The figure shows three views and two pictorial views of one solid part (mm, origin at its lowest corner). Answer the questions. A direction names the side the tool comes from. Coordinates: 2 decimals unless noted, no trailing zeros. Loops run counter-clockwise (first coordinate to the right, second up) from the corner with the lowest first, then second, coordinate; pieces in that order, holes last. Notation, with made-up numbers: M 85.25,68 L 134.25,68 A21 cw 134.25,78 Z; hole C 56,65 d8. An arc over 180 degrees is marked long. One line per item, written item: value. Start each with the question number.
1. The part is cut by section C-C (x = 11.5). Write down the section's boundary in (y, z), then the cut area to 3 significant figures.
2. The part is cut by section B-B (y = 9.5). Write down the section's boundary in (x, z).
3. The part is cut by section A-A (z = 1.45). Write down the section's boundary in (x, y), then the cut area to 3 significant figures.
4. Flat-ended cylindrical pins translate along their axes: pin 1 (2 mm diameter, centred on x = 13.5, z = 4, fed in from +Y); pin 2 (2.5 mm diameter, centred on y = 6.5, z = 3.5, fed in from -X). Find the tip coordinate at first contact, or state that the pin passes through.
5. For the marked faces 1 and 2, determine the directions among +Z, -Z, +X, -X, +Y, -Y from which every point of the face is accessible in a straight line to the end or side of a thin tool.
6. Consider probe 1 along Y at (x, z) = (8, 4.75); probe 2 along X at (y, z) = (3, 2.6); probe 3 along Y at (x, z) = (16, 0.35). Determine where each line is inside the solid, lowest interval first.
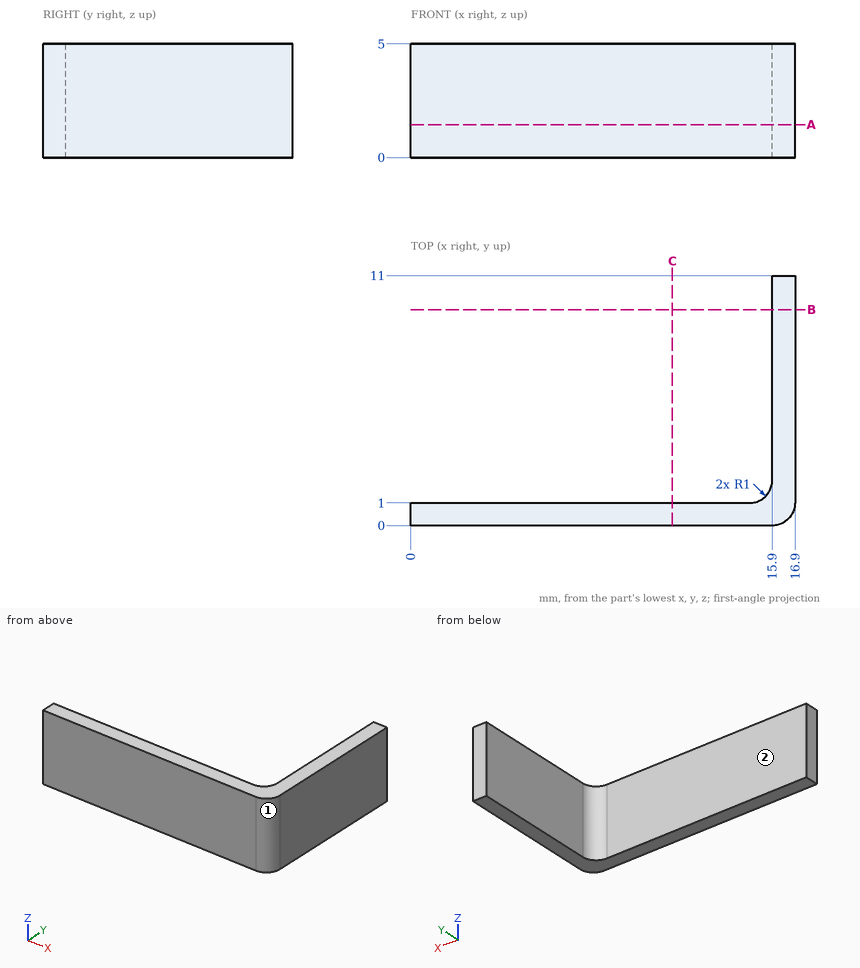
Answer block:
1. outline: M 0,0 L 1,0 L 1,5 L 0,5 Z
1. area: 5.00 mm2
2. outline: M 15.9,0 L 16.9,0 L 16.9,5 L 15.9,5 Z
3. outline: M 0,0 L 15.9,0 A1 ccw 16.9,1 L 16.9,11 L 15.9,11 L 15.9,2 A1 cw 14.9,1 L 0,1 Z
3. area: 26.9 mm2
4. pin 1: stops at y = 1
4. pin 2: stops at x = 15.9
5. face 1: +Z, -Z, +X, -Y
5. face 2: +Z, -Z, -X, +Y
6. probe 1: y = 0 to 1
6. probe 2: x = 15.9 to 16.9
6. probe 3: y = 0.01 to 11
